For this review, take the finished solid that the model builds, in its own axes (mm). A direction names the side the tool comes from. Round coordinates to 2 decimals unless told otherwise and drop trailing zeros. Loops run counter-clockwise (first coordinate to the right, second up) from the corner with the lowest first, then second, coordinate; pieces in that order, holes last.
1) Take a section at D-D (z = 3). State the section outline as (x, y) points.
2) Take a section at A-A (y = -32.5). State the section outline as (x, z) points, then the cut area to 3 significant figures.
3) Wall thickness on L1, parallel to X at y = -21, z = -38; L2, parallel to Z at x = 23.5, y = -7.5; L3, parallel to Y at x = 6, z = -33.5: over which ranges is each line inside the solid? List them lowest first.
4) Take a section at C-C (z = -26). State the section outline as (x, y) points, then the cut area to 3 significant figures.
5) Insertion check: pin 1 (5.5 mm diameter, centred on x = 55.5, y = -44.5, fed in from +Z); pin 2 (5.5 mm diameter, centred on x = 54.5, y = -32.5, fed in from -Z); pin 3 (0.6 mm diameter, centred on x = -2, z = -80, fed in from -Y). Each pin has a flat end and moves straight along its axis. Give the tip position at first contact, or say it passes through.
6) Tool access review of faces 1 (the flat face through (-16.797, -94.4, -29.7)), 2 (the flat face through (18, -8, -79.405)), 3 (the flat face through (-21.877, -36, -31)): name each direction out of +Z, -Z, +X, -X, +Y, -Y from which nothing blocks a thin tool from reaching the whole face with its end or side.
7) Mouldability with a two-part tool opening along Y and no side actions: class faces 4 (the flat face through (-19.337, -50, -30)), 5 (the flat face through (53.043, -94.4, -29.7)), 6 (the flat face through (18, 0, -29)) as pulls with the +Y half, pulls with the -Y half, needs draft (parallel to the pull), parting line crosses it, or undercut.
8) Take a section at B-B (x = 30.5). State the section outline as (y, z) points.
```python
from build123d import *

# Parameters (mm, degrees)
F0_W      = 80
F0_H      = 101.6
F1_DEPTH  = 6.35
F3_DEPTH  = 2.54
F5_DEPTH  = 2.54
F7_DEPTH  = 2.54
F9_DEPTH  = 2.54
F10_W     = 80
F10_H     = 1.27
F11_DEPTH = 2.54
F12_DEPTH = 2.54


with BuildPart() as f1:
    # F0 (on Front) → F1 (new body)
    with BuildSketch(Plane.XZ):
        with Locations((18.1234987736, -29.8747005124)):
            Rectangle(F0_W, F0_H)
    extrude(amount=F1_DEPTH)

    # F2 (on face) → F3 (join)
    with BuildSketch(Plane.YZ.offset(58.1234987736)):
        with BuildLine():
            Line((-93.3970949714, -42.5747005124), (-6.35, -42.5747005124))
            Line((-6.35, -42.5747005124), (-6.35, -29.8747005124))
            Line((-6.35, -29.8747005124), (-6.35, -17.1747005124))
            Line((-6.35, -17.1747005124), (-93.3970949714, -17.1747005124))
            ThreePointArc((-93.3970949714, -17.1747005124), (-95.25, -29.8747005124), (-93.3970949714, -42.5747005124))
        make_face()
    extrude(amount=-F3_DEPTH)

    # F4 (on face) → F5 (join)
    with BuildSketch(Plane(origin=(-21.8765012264, 0, 0), x_dir=(0, -1, 0), z_dir=(-1, 0, 0))):
        with BuildLine():
            Line((93.3970949714, -17.1747005124), (6.35, -17.1747005124))
            Line((6.35, -17.1747005124), (6.35, -42.5747005124))
            Line((6.35, -42.5747005124), (93.3970949714, -42.5747005124))
            ThreePointArc((93.3970949714, -42.5747005124), (95.25, -29.8747005124), (93.3970949714, -17.1747005124))
        make_face()
    extrude(amount=-F5_DEPTH)

    # F6 (on face) → F7 (join)
    with BuildSketch(Plane.YZ.offset(-19.3365012264)):
        with BuildLine():
            ThreePointArc((-95.25, -29.8747005124), (-94.7843345492, -36.2919284389), (-93.3970949714, -42.5747005124))
            Line((-93.3970949714, -42.5747005124), (-92.1396846861, -42.5747005124))
            ThreePointArc((-92.1396846861, -42.5747005124), (-93.5175310216, -36.2910226765), (-93.98, -29.8747005124))
            Line((-93.98, -29.8747005124), (-95.25, -29.8747005124))
        make_face()
        with BuildLine():
            ThreePointArc((-93.3970949714, -17.1747005124), (-94.7843345492, -23.4574725858), (-95.25, -29.8747005124))
            Line((-95.25, -29.8747005124), (-93.98, -29.8747005124))
            ThreePointArc((-93.98, -29.8747005124), (-93.5175310216, -23.4583783483), (-92.1396846861, -17.1747005124))
            Line((-92.1396846861, -17.1747005124), (-93.3970949714, -17.1747005124))
        make_face()
    extrude(amount=F7_DEPTH)

    # F8 (on face) → F9 (join)
    with BuildSketch(Plane(origin=(55.5834987736, 0, 0), x_dir=(0, -1, 0), z_dir=(-1, 0, 0))):
        with BuildLine():
            Line((94.006845472, -29.8747005124), (95.25, -29.8747005124))
            ThreePointArc((95.25, -29.8747005124), (94.7843345492, -23.4574725858), (93.3970949714, -17.1747005124))
            Line((93.3970949714, -17.1747005124), (92.1270949714, -17.1747005124))
            ThreePointArc((92.1270949714, -17.1747005124), (93.5343618687, -23.4555210098), (94.006845472, -29.8747005124))
        make_face()
        with BuildLine():
            ThreePointArc((93.3970949714, -42.5747005124), (94.7843345492, -36.2919284389), (95.25, -29.8747005124))
            Line((95.25, -29.8747005124), (94.006845472, -29.8747005124))
            ThreePointArc((94.006845472, -29.8747005124), (93.5343618687, -36.293880015), (92.1270949714, -42.5747005124))
            Line((92.1270949714, -42.5747005124), (93.3970949714, -42.5747005124))
        make_face()
    extrude(amount=F9_DEPTH)

    # F10 (on face) → F11 (join)
    with BuildSketch(Plane.XZ.offset(6.35)):
        with Locations((18.1234987736, 20.2902994876)):
            Rectangle(F10_W, F10_H)
    extrude(amount=F11_DEPTH)

    # F10 (on face) → F12 (join)
    with BuildSketch(Plane.XZ.offset(6.35)):
        with Locations((18.1234987736, -80.0397005124)):
            Rectangle(F10_W, F10_H)
    extrude(amount=F12_DEPTH)


solid = f1.part
```
Response:
1. outline: (-21.88, -6.35) - (58.12, -6.35) - (58.12, 0) - (-21.88, 0) - close
2. outline: (-21.88, -42.57) - (-19.34, -42.57) - (-19.34, -17.17) - (-21.88, -17.17) - close; (55.58, -42.57) - (58.12, -42.57) - (58.12, -17.17) - (55.58, -17.17) - close
2. area: 129 mm2
3. L1: x = -21.88 to -19.34, 55.58 to 58.12
3. L2: z = -80.67 to -79.4, 19.66 to 20.93
3. L3: y = -6.35 to 0
4. outline: (-21.88, -95.08) - (-16.8, -95.08) - (-16.8, -93.81) - (-19.34, -93.81) - (-19.34, -6.35) - (55.58, -6.35) - (55.58, -93.84) - (53.04, -93.84) - (53.04, -95.08) - (58.12, -95.08) - (58.12, 0) - (-21.88, 0) - close
4. area: 965 mm2
5. pin 1: stops at z = -17.17
5. pin 2: stops at z = -42.57
5. pin 3: stops at y = -8.89
6. face 1: +Z, -Z, -Y
6. face 2: +X, -X, -Y
6. face 3: +Z, -Z, -X, +Y, -Y
7. face 4: undercut
7. face 5: needs draft
7. face 6: pulls with the +Y half
8. outline: (-8.89, -80.67) - (0, -80.67) - (0, 20.93) - (-8.89, 20.93) - (-8.89, 19.66) - (-6.35, 19.66) - (-6.35, -79.4) - (-8.89, -79.4) - close
